```python
from build123d import *

# Parameters (mm, degrees)
F0_W     = 50.8
F0_H     = 76.2
F1_DEPTH = 6.35
F3_D     = 28.5623
F5_D     = 5.1054
F6_R     = 5.08


with BuildPart() as f1:
    # F0 (on Front) → F1 (new body)
    with BuildSketch(Plane.XZ):
        Polygon((-67.407699, 49.186888), (-80.107699, 0), (-29.307699, 0), (-16.607699, 49.186888), align=None)
        with Locations((-54.707699, -38.1)):
            Rectangle(F0_W, F0_H)
    extrude(amount=F1_DEPTH)

    # F3 (through all)
    with Locations(Plane.XZ.offset(6.35)):
        with Locations((-46.160249, 22.205738), (-51.269072, -15.550187), (-54.429126, -53.518912)):
            Hole(F3_D / 2)

    # F5 (through all)
    with Locations(Plane.XZ.offset(6.35)):
        with Locations((-36.903126, -35.992912), (-36.903126, -71.044912), (-71.955126, -71.044912), (-71.955126, -35.992912)):
            Hole(F5_D / 2)

    # F6
    f6_edges = [f1.edges().sort_by_distance(p)[0] for p in [
        (-67.407699, -3.175, 49.186888),
        (-16.607699, -3.175, 49.186888),
        (-80.107699, -3.175, 0),
        (-80.107699, -3.175, -76.2),
        (-29.307699, -3.175, -76.2),
        (-29.307699, -3.175, 0),
    ]]
    fillet(f6_edges, radius=F6_R)


solid = f1.part
```
Check sheet for the modelled part. Datum: model origin and axes. Units: mm. A direction names the side the tool comes from. Give positions to 0.01 mm unless a question says otherwise; leave off trailing zeros. Order: outer loops, then holes, each group sorted by start corner. A loop starts at its lowest first (then second) coordinate and runs counter-clockwise, first axis right, second up. Notation, with made-up numbers: M -19,3 L 7,3 A11 ccw 7,18 Z; hole C 59,44 d7. An arc over 180 degrees is marked long. Answer in a Markdown table with one row per item. Add a question column.
Q1. Access from +Z, -Z, +X, -X, +Y, -Y to the whole of each face (thin tool, end or side, straight path). Record for faces 1 (the flat face through (-29.308, -3, -36)), 2 (the cylindrical face through (-78.66, -3.22, -74.67)).
Q2. Gauge pin test, flat ends, axial feed: pin 1 Ø4.5 at (x, z) = (-36.9, -35.99) entering from +Y; pin 2 Ø1.9 at (y, z) = (-2.5, -38) entering from +X. Record the tip position at first contact, or that the pin passes through.
Q3. Sectioned sample at B-B, the plane x = -57.5. Record the boundary of the cut face in (y, z), and give its area (3 significant figures).
Q4. Sectioned sample at C-C, the plane y = -4. Record the boundary of the cut face in (x, z), and give its area (3 significant figures).
Q5. Sectioned sample at A-A, the plane z = 33. Record the boundary of the cut face in (x, y), and give its area (3 significant figures).
Q6. Sectioned sample at D-D, the plane z = -32. Record the boundary of the cut face in (x, y).
Q7. Release check for a two-part mould opening along Z. For faces 3 (the cylindrical face through (-69.405, -3.131, -70.933)), 4 (the flat face through (-74.09, -3.13, 23.31)), 5 (the flat face through (-55, -3, -76.2)) record: released by +Z, released by -Z, zero draft, split by the parting line, or undercut.
Q8. Thickness scan on L1, parallel to X at y = -4, z = -70.5; L2, parallel to Z at x = -59, y = -0.25; L3, parallel to X at y = -0.25, z = 24. Record the ranges inside material, lowest first.
Verdict:
| question | item | result |
|---|---|---|
| 1 | face 1 | -Z, +X, +Y, -Y |
| 1 | face 2 | -Z, -X, +Y, -Y |
| 2 | pin 1 | through |
| 2 | pin 2 | x = -29.31 |
| 3 | outline | M -6.35,-76.2 L 0,-76.2 L 0,-67.47 L -6.35,-67.47 Z; M -6.35,-39.57 L 0,-39.57 L 0,-28.4 L -6.35,-28.4 Z; M -6.35,-2.7 L 0,-2.7 L 0,13.52 L -6.35,13.52 Z; M -6.35,30.89 L 0,30.89 L 0,49.19 L -6.35,49.19 Z |
| 3 | area | 346 mm² |
| 4 | outline | M -80.11,-71.12 A5.08 ccw -75.03,-76.2 L -34.39,-76.2 A5.08 ccw -29.31,-71.12 L -29.31,-0.65 A5.08 cw -29.15,0.62 L -18.25,42.84 A5.08 ccw -23.17,49.19 L -63.47,49.19 A5.08 ccw -68.39,45.38 L -79.95,0.62 A5.08 ccw -80.11,-0.65 Z; hole C -71.96,-71.04 d5.11; hole C -71.96,-35.99 d5.11; hole C -54.43,-53.52 d28.56; hole C -51.27,-15.55 d28.56; hole C -46.16,22.21 d28.56; hole C -36.9,-71.04 d5.11; hole C -36.9,-35.99 d5.11 |
| 4 | area | 4,340 mm² |
| 5 | outline | M -71.59,-6.35 L -55.51,-6.35 L -55.51,0 L -71.59,0 Z; M -36.81,-6.35 L -20.79,-6.35 L -20.79,0 L -36.81,0 Z |
| 5 | area | 204 mm² |
| 6 | outline | M -80.11,-6.35 L -29.31,-6.35 L -29.31,0 L -80.11,0 Z |
| 7 | face 3 | undercut |
| 7 | face 4 | released by +Z |
| 7 | face 5 | released by -Z |
| 8 | L1 | -80.11 to -74.45, -69.46 to -39.4, -34.41 to -29.31 |
| 8 | L2 | -76.2 to -67.05, -39.99 to -27.56, -3.54 to 15.95, 28.46 to 49.19 |
| 8 | L3 | -73.91 to -60.33, -31.99 to -23.11 |
